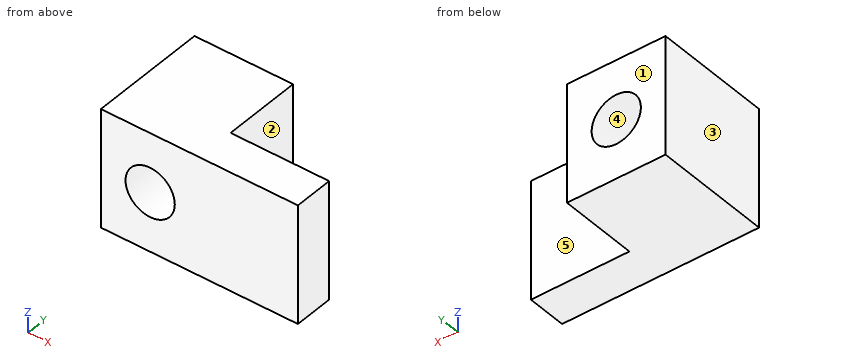
Autodesk Inventor part; units mm, degrees
ref_plane "YZ Plane" through (0, 0, 0) normal (1, 0, 0) x (0, 1, 0)
ref_plane "XZ Plane" through (0, 0, 0) normal (0, 1, 0) x (-1, 0, 0)
ref_plane "XY Plane" through (0, 0, 0) normal (0, 0, 1) x (1, 0, 0)
sketch "Sketch1" plane through (0, 0, 0) normal (0, 0, 1) x (1, 0, 0)
  line L0 (0, 0) -> (127, 0)
  line L1 (127, 0) -> (127, 25.3956)
  line L2 (127, 25.3956) -> (63.5, 25.3956)
  line L3 (63.5, 25.3956) -> (63.5, 76.2)
  line L4 (63.5, 76.2) -> (0, 76.2)
  line L5 (0, 76.2) -> (0, 0)
  dimension "d0" = 127
  dimension "d16" = 63.5
  dimension "d17" = 25.3956
  dimension "d18" = 76.2
extrude "Extrusion1" add sketch "Sketch1" along normal blind 76.2
sketch "Sketch2" plane through (0, 76.2, 0) normal (0, 1, 0) x (1, 0, 0)
  circle A0 centre (31.75, -38.1) radius 15.875
  dimension "d3" = 31.75
extrude "Extrusion2" cut sketch "Sketch2" against normal through all
properties part number "SamplePart"
Geometry check sheet. Reference: the model listing, model coordinates, mm. Face numbers are marked on the shaded views. A direction names the side the tool comes from. Give positions to 0.01 mm unless a question says otherwise; leave off trailing zeros. Order: outer loops, then holes, each group sorted by start corner. A loop starts at its lowest first (then second) coordinate and runs counter-clockwise, first axis right, second up.
1. Section check C-C, the plane y = 13. Enter the section's corners in (x, z) (3 decimals), and give its area (3 significant figures).
2. Section check B-B, the plane z = 38.1. Enter the section's corners in (x, y) (3 decimals).
3. Access from +Z, -Z, +X, -X, +Y, -Y to the whole of each face (thin tool, end or side, straight path). Record for the marked faces 1 and 2.
4. Section check A-A, the plane x = 31.75. Enter the section's corners in (y, z) (3 decimals), and give its area (3 significant figures).
5. Section check D-D, the plane z = 12.5. Enter the section's corners in (x, y), and give its area (3 significant figures).
6. Release check for a two-part mould opening along X. For the marked faces 3, 4 and 5 record: pulls with the +X half, pulls with the -X half, needs draft (parallel to the pull), parting line crosses it, or undercut.
7. Gauge pin test, flat ends, axial feed: pin 1 Ø8 at (y, z) = (29.5, 62.5) entering from +X; pin 2 Ø4 at (x, z) = (27.5, 52.5) entering from -Y; pin 3 Ø1.5 at (x, z) = (70, 36) entering from +Y. Record the tip position at first contact, or that the pin passes through.
8. Thickness scan on L1, parallel to X at y = 57, z = 38.1 (3 decimals); L2, parallel to Z at x = 31.75, y = 49 (3 decimals); L3, parallel to Y at x = 66, z = 65. Record the ranges inside material, lowest first.
Values follow:
1. outline: (0, 0) - (127, 0) - (127, 76.2) - (0, 76.2) - close; hole circle Ø31.75 at (31.75, 38.1)
1. area: 8,890 mm2
2. outline: (0, 0) - (15.875, 0) - (15.875, 76.2) - (0, 76.2) - close; (47.625, 0) - (127, 0) - (127, 25.396) - (63.5, 25.396) - (63.5, 76.2) - (47.625, 76.2) - close
3. face 1: +Z, -Z, +X, -X, +Y
3. face 2: +Z, -Z, +X, +Y
4. outline: (0, 0) - (76.2, 0) - (76.2, 22.225) - (0, 22.225) - close; (0, 53.975) - (76.2, 53.975) - (76.2, 76.2) - (0, 76.2) - close
4. area: 3,390 mm2
5. outline: (0, 0) - (127, 0) - (127, 25.4) - (63.5, 25.4) - (63.5, 76.2) - (0, 76.2) - close
5. area: 6,450 mm2
6. face 3: pulls with the -X half
6. face 4: undercut
6. face 5: needs draft
7. pin 1: stops at x = 63.5
7. pin 2: stops at y = 0
7. pin 3: stops at y = 25.4
8. L1: x = 0 to 15.875, 47.625 to 63.5
8. L2: z = 0 to 22.225, 53.975 to 76.2
8. L3: y = 0 to 25.4
